The model under review builds one solid part; all positions refer to its coordinate system, in mm. A direction names the side the tool comes from. Coordinates: 2 decimals unless noted, no trailing zeros. Loops run counter-clockwise (first coordinate to the right, second up) from the corner with the lowest first, then second, coordinate; pieces in that order, holes last. Notation, with made-up numbers: M 81.25,-27.5 L 103.25,-27.5 A10 ccw 103.25,-8.5 Z; hole C 31,-14 d2. An arc over 180 degrees is marked long. Use CSV: the item, a comma, the result in double quotes. Start each with the question number.
from build123d import *

# Parameters (mm, degrees)
SKETCH1_R               = 20
SKETCH1_R_2             = 7.5
BOSS_EXTRUDE1_DEPTH     = 6
SKETCH2_R               = 12
SKETCH2_R_2             = 7.5
BOSS_EXTRUDE2_DEPTH     = 14
CUT_EXTRUDE1_DEPTH      = 35.641016151
CUT_EXTRUDE1_DEPTH_BACK = 35.641016151
SKETCH3_R               = 1.5
SKETCH4_R               = 18
SKETCH4_R_2             = 7.5
BOSS_EXTRUDE3_DEPTH     = 6
BOSS_EXTRUDE4_START     = -6
SKETCH5_R               = 1.75
BOSS_EXTRUDE4_DEPTH     = 6
CUT_EXTRUDE2_DEPTH      = 42.39519906
CUT_EXTRUDE2_DEPTH_BACK = 6
SKETCH6_R               = 2
SKETCH7_R               = 8
CUT_EXTRUDE3_DEPTH      = 2


with BuildPart() as part:
    # Sketch1 → Boss-Extrude1 (new body)
    with BuildSketch(Plane(origin=(0, 0, 0), x_dir=(1, 0, 0), z_dir=(0, 1, 0))):
        with Locations(Location((0, 0, 0), (0, 0, 270))):
            Circle(SKETCH1_R)
        with Locations(Location((0, 0, 0), (0, 0, 270))):
            Circle(SKETCH1_R_2, mode=Mode.SUBTRACT)
    extrude(amount=BOSS_EXTRUDE1_DEPTH)

    # Sketch2 → Boss-Extrude2 (add)
    with BuildSketch(Plane(origin=(0, 6, 0), x_dir=(1, 0, 0), z_dir=(0, 1, 0))):
        with Locations(Location((0, 0.535416774, 0), (0, 0, 270))):
            Circle(SKETCH2_R)
        with Locations(Location((0, 0, 0), (0, 0, 270))):
            Circle(SKETCH2_R_2, mode=Mode.SUBTRACT)
    extrude(amount=BOSS_EXTRUDE2_DEPTH)

    # Sketch3 → Cut-Extrude1 (cut, two sides: drawn at the far end of the back side and taken through both)
    with BuildSketch(Plane.XY.offset(-CUT_EXTRUDE1_DEPTH_BACK)):
        with Locations((0, 9)):
            Circle(SKETCH3_R)
    extrude(amount=CUT_EXTRUDE1_DEPTH + CUT_EXTRUDE1_DEPTH_BACK, mode=Mode.SUBTRACT)

    # Sketch4 → Boss-Extrude3 (add)
    with BuildSketch(Plane(origin=(0, 20, 0), x_dir=(1, 0, 0), z_dir=(0, 1, 0))):
        with Locations(Location((0, 0, 0), (0, 0, 270))):
            Circle(SKETCH4_R)
        with Locations(Location((0, 0, 0), (0, 0, 270))):
            Circle(SKETCH4_R_2, mode=Mode.SUBTRACT)
    extrude(amount=BOSS_EXTRUDE3_DEPTH)

    # Sketch5 → Boss-Extrude4 (add)
    # profile 1 of 2: a face of its own
    with BuildSketch(Plane(origin=(0, 26, 0), x_dir=(1, 0, 0), z_dir=(0, 1, 0)).offset(BOSS_EXTRUDE4_START)):
        with BuildLine():
            Line((-23.358800107, 2.984171955), (-16.970562748, 6))
            ThreePointArc((-16.970562748, 6), (-18, 0), (-16.970562748, -6))
            Line((-16.970562748, -6), (-23.358800107, -2.984171955))
            ThreePointArc((-23.358800107, -2.984171955), (-25.25, 0), (-23.358800107, 2.984171955))
        make_face()
        with Locations(Location((-21.95, 0, 0), (0, 0, 270))):
            Circle(SKETCH5_R, mode=Mode.SUBTRACT)
    # profile 2 of 2: a face of its own
    with BuildSketch(Plane(origin=(0, 26, 0), x_dir=(1, 0, 0), z_dir=(0, 1, 0)).offset(BOSS_EXTRUDE4_START)):
        with BuildLine():
            Line((23.358800107, 2.984171955), (16.970562748, 6))
            ThreePointArc((16.970562748, 6), (18, 0), (16.970562748, -6))
            Line((16.970562748, -6), (23.358800107, -2.984171955))
            ThreePointArc((23.358800107, -2.984171955), (25.25, 0), (23.358800107, 2.984171955))
        make_face()
        with Locations(Location((21.95, 0, 0), (0, 0, 270))):
            Circle(SKETCH5_R, mode=Mode.SUBTRACT)
    extrude(amount=BOSS_EXTRUDE4_DEPTH)

    # Sketch6 → Cut-Extrude2 (cut, two sides: drawn at the far end of the back side and taken through both)
    with BuildSketch(Plane.XZ.offset(-CUT_EXTRUDE2_DEPTH_BACK)):
        with Locations(Location((-10.606601718, 10.606601718, 0), (0, 0, 270))):
            Circle(SKETCH6_R)
        with Locations(Location((10.606601718, 10.606601718, 0), (0, 0, 270))):
            Circle(SKETCH6_R)
        with Locations(Location((10.606601718, -10.606601718, 0), (0, 0, 270))):
            Circle(SKETCH6_R)
        with Locations(Location((-10.606601718, -10.606601718, 0), (0, 0, 270))):
            Circle(SKETCH6_R)
    extrude(amount=CUT_EXTRUDE2_DEPTH + CUT_EXTRUDE2_DEPTH_BACK, mode=Mode.SUBTRACT)

    # Sketch7 → Cut-Extrude3 (cut)
    with BuildSketch(Plane(origin=(0, 26, 0), x_dir=(1, 0, 0), z_dir=(0, 1, 0))):
        with Locations(Location((0, 0, 0), (0, 0, 270))):
            Circle(SKETCH7_R)
    extrude(amount=-CUT_EXTRUDE3_DEPTH, mode=Mode.SUBTRACT)


solid = part.part
1. Add section D-D (x = 21.95). Write out the cut boundary in (y, z).
2. For faces 5 (the cylindrical face through (0, 23, -18)), 6 (the flat face through (-7.4, 20, 9.2)), 7 (the cylindrical face through (-7.81, 25.01, -1.73)), list the 3-axis set-ups (+Z, -Z, +X, -X, +Y, -Y) from which the entire face can be reached by the end or side of a thin tool; tool diameter is ignored.
3. To check wall thickness, follow line 1 along Y through (x, z) = (-15, -9); line 2 along X through (y, z) = (13, 0); line 3 along Y through (x, z) = (6, 18). State the ranges of each line that lie inside material, in increasing order.
4. Draft analysis for pull direction Y (two halves, no side actions). For faces 1 (the cylindrical face through (-0.325, 7.536, 9.378)), 2 (the flat face through (0.4, 26, -8.3)), 3 (the cylindrical face through (23.685, 22.958, -0.228)), 4 (the cylindrical face through (3.6, 12.9, 10.91)), state which applies: released by +Y, released by -Y, zero draft, split by the parting line, or undercut.
5. Add section A-A (x = 0). Write out the cut boundary in (y, z).
6. Add section C-C (y = 9). Write out the cut boundary in (x, z), plus the area to 3 significant figures.
7. Insertion check: pin 1 Ø3 at (x, z) = (21.95, 0) entering from +Y; pin 2 Ø5 at (y, z) = (9, -13.5) entering from -X; pin 3 Ø10 at (y, z) = (5.5, 2.5) entering from -X; pin 4 Ø4 at (x, y) = (-3.5, 16) entering from -Z. Each pin has a flat end and moves straight along its axis. Give the tip position at first contact, or say it passes through.
8. Add section B-B (z = -1). Write out the cut boundary in (x, y).
Solved:
1,outline,"M 20,-3.65 L 26,-3.65 L 26,-1.75 L 20,-1.75 Z; M 20,1.75 L 26,1.75 L 26,3.65 L 20,3.65 Z"
2,face 5,"-Z, +Y"
2,face 6,"none"
2,face 7,"+Y"
3,line 1,"y = 0 to 6, 20 to 26"
3,line 2,"x = -11.99 to -7.5, 7.5 to 11.99"
3,line 3,"y = 0 to 6"
4,face 1,"undercut"
4,face 2,"released by +Y"
4,face 3,"zero draft"
4,face 4,"undercut"
5,outline,"M 0,-20 L 6,-20 L 6,-12.54 L 7.5,-12.54 L 7.5,-7.5 L 0,-7.5 Z; M 0,7.5 L 7.5,7.5 L 7.5,11.46 L 6,11.46 L 6,20 L 0,20 Z; M 10.5,-12.54 L 20,-12.54 L 20,-18 L 26,-18 L 26,-8 L 24,-8 L 24,-7.5 L 10.5,-7.5 Z; M 10.5,7.5 L 24,7.5 L 24,8 L 26,8 L 26,18 L 20,18 L 20,11.46 L 10.5,11.46 Z"
6,outline,"M -1.5,-12.44 L -1.5,-7.35 A7.5 cw -1.5,7.35 L -1.5,11.37 A12 ccw Z; M 1.5,-12.44 A12 ccw 1.5,11.37 L 1.5,7.35 A7.5 cw 1.5,-7.35 Z"
6,area,"249 mm^2"
7,pin 1,"passes through"
7,pin 2,"stops at x = -5.87"
7,pin 3,"stops at x = -20"
7,pin 4,"stops at z = -12.44"
8,outline,"M -25.09,20 L -23.39,20 L -23.39,26 L -25.09,26 Z; M -20.51,20 L -11.99,20 L -11.99,6 L -19.97,6 L -19.97,0 L -7.43,0 L -7.43,24 L -7.94,24 L -7.94,26 L -20.51,26 Z; M 7.43,0 L 19.97,0 L 19.97,6 L 11.99,6 L 11.99,20 L 20.51,20 L 20.51,26 L 7.94,26 L 7.94,24 L 7.43,24 Z; M 23.39,20 L 25.09,20 L 25.09,26 L 23.39,26 Z"
